```python
from build123d import *

# Parameters (mm, degrees)
F2_R = 6.35


with BuildPart() as f3:
    # F3: sweep along a path in F0
    with BuildLine(Plane.XZ) as f3_path:
        Line((0, 0), (0, 88.9))
        ThreePointArc((0, 88.9), (-6.35, 99.8985226281), (-19.05, 99.8985226281))
        Line((-19.05, 99.8985226281), (-76.1846965395, 66.9117902009))
        ThreePointArc((-76.1846965395, 66.9117902009), (-82.1019545334, 52.6262657001), (-69.8346965395, 43.2132675729))
        Line((-69.8346965395, 43.2132675729), (-50.8, 43.2132675729))
        ThreePointArc((-50.8, 43.2132675729), (-41.8197438789, 39.4935236939), (-38.1, 30.5132675729))
        Line((-38.1, 30.5132675729), (-38.1, 0))
    # F2 (on line) → F3 (sweep)
    with BuildSketch(Plane.XY):
        Circle(F2_R)
    sweep(path=f3_path.line)


solid = f3.part
```
Check sheet for the modelled part. Datum: model origin and axes. Units: mm. A direction names the side the tool comes from. Coordinates: 2 decimals unless noted, no trailing zeros. Write each loop counter-clockwise with the first axis right and the second up, starting at its lowest first coordinate (ties: lowest second). Pieces come first, ordered by that corner, then holes. Notation, with made-up numbers: (45, 43.25) - (49, 43.25) arc R16 ccw to (49, 60.25) - close; hole circle Ø11 at (85.25, -11.5). An arc over 180 degrees is marked (long way). One line per question, with ' | ' between items.
Item 1: Thickness scan on line 1 (Y direction, x = -36.5, z = 89.5); line 2 (Z direction, x = -76, y = -4.5); line 3 (X direction, y = -5, z = 16.5). Record the ranges inside material, lowest first. Write a range as [from, to].
Determined:
line 1: y = [-6.34, 6.34] | line 2: z = [39.88, 50.48], [61.35, 72.19] | line 3: x = [-42.01, -34.19], [-3.91, 3.91]
Item 2: Gauge pin test, flat ends, axial feed: P1, Ø3, axis at x = -6, z = 86.5, coming from the +Y side; P2, Ø1.5, axis at x = -35.5, y = -3, coming from the +Z side; P3, Ø6, axis at y = -0.5, z = 29, coming from the -X side. Record the tip position at first contact, or that the pin passes through.
Determined:
P1: stops at y = 4.48 | P2: stops at z = 97.46 | P3: stops at x = -44.62
Item 3: Mould release check, pull along Z, two halves, no side actions. Record for faces 1 (the face through (-31.756, 0.279, 15.043)), 2 (the face through (0, 0, 0)), 3 (the face through (-60.184, 1.907, 37.156)): pulls with the +Z half, pulls with the -Z half, needs draft (parallel to the pull), parting line crosses it, or undercut.
Determined:
face 1: needs draft | face 2: pulls with the -Z half | face 3: undercut
Item 4: Access from +Z, -Z, +X, -X, +Y, -Y to the whole of each face (thin tool, end or side, straight path). Record for faces 4 (the face through (-1.38, -6.2, 45.07)), 5 (the face through (-51.046, 1.907, 88.42)).
Determined:
face 4: -Z | face 5: none
Item 5: Sectioned sample at A-A on y = 4.25. Record the boundary of the cut face in (x, z), plus the area to 3 significant figures.
Determined:
outline: (-78.54, 71) arc R17.42 ccw to (-69.83, 38.5) - (-50.8, 38.5) arc R7.98 cw to (-42.82, 30.51) - (-42.82, 0) - (-33.38, 0) - (-33.38, 30.51) arc R17.42 ccw to (-50.8, 47.93) - (-69.83, 47.93) arc R7.98 cw to (-73.83, 62.83) - (-16.69, 95.81) arc R7.98 cw to (-4.72, 88.9) - (-4.72, 0) - (4.72, 0) - (4.72, 88.9) arc R17.42 ccw to (-21.41, 103.98) - close | area: 2,680 mm2
